Autodesk Inventor part; units mm, degrees
ref_plane "YZ Plane" through (0, 0, 0) normal (1, 0, 0) x (0, 1, 0)
ref_plane "XZ Plane" through (0, 0, 0) normal (0, 1, 0) x (-1, 0, 0)
ref_plane "XY Plane" through (0, 0, 0) normal (0, 0, 1) x (1, 0, 0)
sketch "Sketch1" plane through (0, 0, 0) normal (0, 1, 0) x (-1, 0, 0)
  line L0 (-60, 120) -> (60, 120)
  line L1 (60, 120) -> (60, -110)
  line L2 (50, -120) -> (-50, -120)
  line L3 (-60, -110) -> (-60, 120)
  line L4 (-60, 120) -> (60, -120) construction
  line L5 (60, 120) -> (-60, -120) construction
  line L6 (-60, 120) -> (60, 120)
  line L7 (60, 120) -> (60, 0)
  line L8 (60, 0) -> (-60, 0)
  line L9 (-60, 0) -> (-60, 120)
  line L10 (60, 0) -> (-60, 120) construction
  line L11 (-60, 0) -> (60, 120) construction
  circle A0 centre (0, 60) radius 54
  line L12 (54, 60) -> (60, 60) construction
  arc A1 (50, -120) -> (60, -110) centre (50, -110) ccw
  arc A2 (-60, -110) -> (-50, -120) centre (-50, -110) ccw
  point P0 (0, 0)
  dimension "d0" = 120
  dimension "d1" = 240
  dimension "d2" = 120
  dimension "d3" = 6
  dimension "d4" = 10
extrude "Extrusion1" add sketch "Sketch1" along normal blind 6
sketch "Sketch2" plane through (0, 0, 0) normal (0, -1, 0) x (1, 0, 0)
  circle A0 centre (0, 60) radius 54 construction
  line L0 (60, 120) -> (60, -110)
  line L1 (-60, 120) -> (60, 120)
  line L2 (-60, -110) -> (-60, 120)
  arc A1 (-60, -110) -> (-50, -120) centre (-50, -110) ccw
  line L3 (50, -120) -> (-50, -120)
  arc A2 (50, -120) -> (60, -110) centre (50, -110) ccw
  line L4 (57, -110) -> (57, 117)
  line L5 (57, 117) -> (-57, 117)
  line L6 (-57, 117) -> (-57, -110)
  arc A3 (-57, -110) -> (-50, -117) centre (-50, -110) ccw
  line L7 (-50, -117) -> (50, -117)
  arc A4 (50, -117) -> (57, -110) centre (50, -110) ccw
  line L8 (57, 117) -> (57, 120)
  line L9 (-57, 117) -> (-57, 120)
  point P0 (0, 0)
  dimension "d7" = 3
extrude "Extrusion2" add sketch "Sketch2" along normal blind 15 contours L0 A2 L3 A1 L2 L1 L9 L6 A3 L7 A4 L4 L8
sketch "Sketch3" plane through (0, -15, 0) normal (0, -1, 0) x (1, 0, 0)
  line L0 (60, -110) -> (60, 120)
  line L1 (60, 120) -> (57, 120)
  line L2 (57, 120) -> (57, -110)
  arc A0 (50, -117) -> (57, -110) centre (50, -110) ccw
  line L3 (50, -117) -> (-50, -117)
  arc A1 (-57, -110) -> (-50, -117) centre (-50, -110) ccw
  line L4 (-57, -110) -> (-57, 120)
  line L5 (-57, 120) -> (-60, 120)
  line L6 (-60, 120) -> (-60, -110)
  arc A2 (-60, -110) -> (-50, -120) centre (-50, -110) ccw
  line L7 (-50, -120) -> (50, -120)
  arc A3 (50, -120) -> (60, -110) centre (50, -110) ccw
  line L8 (57, 120) -> (54, 120)
  line L9 (-60, 120) -> (60, 120) construction
  line L10 (54, 120) -> (54, -110)
  line L11 (50, -114) -> (25, -114)
  arc A4 (50, -114) -> (54, -110) centre (50, -110) ccw
  line L12 (0, 0) -> (0, -136) construction
  line L13 (-57, 120) -> (-54, 120)
  line L14 (-54, 120) -> (-54, -110)
  line L15 (-50, -114) -> (25, -114)
  arc A5 (-54, -110) -> (-50, -114) centre (-50, -110) ccw
  dimension "d10" = 3
extrude "Extrusion3" add sketch "Sketch3" along normal blind 6
sketch "Sketch5" plane through (0, 6, 0) normal (0, 1, 0) x (1, 0, 0)
  circle A0 centre (0, -60) radius 54
  line L0 (60, -120) -> (60, 110)
  arc A1 (60, 110) -> (50, 120) centre (50, 110) ccw
  line L1 (50, 120) -> (-50, 120)
  arc A2 (-50, 120) -> (-60, 110) centre (-50, 110) ccw
  line L2 (-60, 110) -> (-60, -120)
  line L3 (-60, -120) -> (60, -120)
  line L4 (-67.6504, 0) -> (67.3496, 0) construction
  circle A3 centre (0, 60) radius 54
  point P0 (0, 0)
extrude "Extrusion4" cut sketch "Sketch5" against normal up to next contours A3
sketch "Sketch6" plane through (0, 6, 0) normal (0, 1, 0) x (1, 0, 0)
  circle A0 centre (0, -60) radius 54
  circle A1 centre (0, 60) radius 54
  circle A2 centre (0, 60) radius 54
  circle A3 centre (0, -60) radius 54
  line L0 (60, -120) -> (60, 110)
  arc A4 (60, 110) -> (50, 120) centre (50, 110) ccw
  line L1 (50, 120) -> (-50, 120)
  arc A5 (-50, 120) -> (-60, 110) centre (-50, 110) ccw
  line L2 (-60, 110) -> (-60, -120)
  line L3 (-60, -120) -> (60, -120)
  line L4 (-50.0326, 0) -> (43.9674, 0) construction
  line L5 (0, -60) -> (-70, -60) construction
  line L6 (0, -60) -> (0, -118) construction
  point P0 (0, 0)
  point P1 (-51, -9)
  point P2 (-51, -111)
  point P3 (51, -9)
  point P4 (51, -111)
  point P5 (-51, 9)
  point P6 (-51, 111)
  point P7 (51, 111)
  point P8 (51, 9)
  dimension "d15" = 18
  dimension "d16" = 9
hole "Hole1" at (-51, 6, 9) at (-51, 6, 111) at (51, 6, 111) at (51, 6, 9) at (-51, 6, -111) at (-51, 6, -9) at (51, 6, -111) at (51, 6, -9) direction (0, -1, 0) diameter 3.1 end through all
sketch "Sketch7" plane through (0, -21, 0) normal (0, -1, 0) x (1, 0, 0)
  line L0 (57, 120) -> (57, -110) construction
  line L1 (57, -110) -> (57, 120)
  line L2 (-57, -110) -> (-57, 120) construction
  line L3 (-57, 120) -> (-57, -110)
  line L4 (57, 120) -> (57, -110)
  line L5 (0, 119) -> (0, 0) construction
  point P0 (57, 60)
  point P1 (57, -60)
  point P2 (57, 114)
  point P3 (-57, 114)
  point P4 (-57, 102)
  point P5 (57, 102)
  point P6 (-57, 90)
  point P7 (57, 90)
  point P8 (-57, 78)
  point P9 (57, 78)
  point P10 (-57, 66)
  point P11 (57, 66)
  point P12 (-57, 54)
  point P13 (57, 54)
  point P14 (-57, 42)
  point P15 (57, 42)
  point P16 (-57, 30)
  point P17 (57, 30)
  point P18 (-57, 18)
  point P19 (57, 18)
  point P20 (-57, 6)
  point P21 (57, 6)
  point P22 (-57, -6)
  point P23 (57, -6)
  point P24 (-57, -18)
  point P25 (57, -18)
  point P26 (-57, -30)
  point P27 (57, -30)
  point P28 (-57, -42)
  point P29 (57, -42)
  point P30 (-57, -54)
  point P31 (57, -54)
  point P32 (-57, -66)
  point P33 (57, -66)
  dimension "d24" = 6
  dimension "d27" = 12
hole "Hole2" at (57, -21, 114) at (-57, -21, 114) at (-57, -21, 102) at (57, -21, 102) at (-57, -21, 90) at (57, -21, 90) at (-57, -21, 78) at (57, -21, 78) at (-57, -21, 66) at (57, -21, 66) at (-57, -21, 54) at (57, -21, 54) at (-57, -21, 42) at (57, -21, 42) at (-57, -21, 30) at (57, -21, 30) at (-57, -21, 18) at (57, -21, 18) at (-57, -21, 6) at (57, -21, 6) at (-57, -21, -6) at (57, -21, -6) at (-57, -21, -18) at (57, -21, -18) at (-57, -21, -30) at (57, -21, -30) at (-57, -21, -42) at (57, -21, -42) at (-57, -21, -54) at (57, -21, -54) at (-57, -21, -66) at (57, -21, -66) direction (0, 1, 0) diameter 3.1 depth 4 tip angle 118
equation "\"d0\" = hull_width"
equation "\"d1\" = hull_length"
equation "\"d2\" = hull_width"
equation "\"d3\" = 2 * thickness"
equation "\"d4\" = roundness"
equation "\"d5\" = 2 * thickness"
equation "\"d7\" = thickness"
equation "\"d8\" = 5 * thickness"
equation "\"d10\" = thickness"
equation "\"d11\" = 2 * thickness"
equation "\"d13\" = 2 * thickness"
equation "\"d22\" = 1.33333 * thickness"
equation "\"d37\" = 1.33333 * thickness"
equation "\"thickness\" = 3"
equation "\"roundness\" = 10"
equation "\"hull_width\" = 120"
equation "\"hull_length\" = 2 * hull_width"
properties part number "Cup_Dispenser_Hull"
Here's how the part is built. I have some questions about the finished solid (model axes, mm). A direction names the side the tool comes from. Round coordinates to 2 decimals unless told otherwise and drop trailing zeros. Order: outer loops, then holes, each group sorted by start corner. A loop starts at its lowest first (then second) coordinate and runs counter-clockwise, first axis right, second up. Notation, with made-up numbers: (-29, 31.5) -> (0, 31.5) arc R29 ccw to (0, 63.5) -> close; hole circle Ø9 at (24, 50.5). An arc over 180 degrees is marked (long way). Use a Markdown table: item, result. Add a question column.
(1) For faces 4 (the face through (-57, -7, 3)), 5 (the face through (-56.99, -7.31, -117.15)), 6 (the face through (-54, -18, 7)), which set-ups out of +Z, -Z, +X, -X, +Y, -Y let a thin tool reach every point of the face, with its end or its side?
(2) Suppose I cut it at C-C, the plane x = -16. Please give me the cut outline in (y, z), and give its area (3 significant figures).
(3) Suppose I cut it at A-A, the plane x = 35. Please give me the cut outline in (y, z), and give its area (3 significant figures).
(4) Suppose I cut it at B-B, the plane y = -9.75. Please give me the cut outline in (x, z), and give its area (3 significant figures).
(5) I need wall thicknesses on line 1 along X through (y, z) = (-20, -54); line 2 along X through (y, z) = (-12.5, 65); line 3 along X through (y, z) = (-19.5, 3). Which ranges of each line are inside material? Lowest first, please.
(6) For pin 1 Ø3.5 at (x, z) = (-51, 9) entering from -Y; pin 2 Ø1.5 at (x, y) = (-3, -6) entering from +Z; pin 3 Ø1.9 at (x, z) = (51, 9) entering from -Y; pin 4 Ø2.5 at (x, z) = (-57, 90) entering from -Y, each with a flat end and sliding along its axis, tell me the tip position at first contact or that it passes through.
(7) If we mould it in two halves opening along X, with no side actions, what happens to faces 1 (the face through (1, -7, -120)), 2 (the face through (57.15, -7.31, -116.99)), 3 (the face through (-54.9, -7.4, -115))? For each: released by +X, released by -X, zero draft, split by the parting line, or undercut.
Verdict:
| question | item | result |
|---|---|---|
| 1 | face 4 | +Z |
| 1 | face 5 | -Z, -X, +Y, -Y |
| 1 | face 6 | +Z, -Y |
| 2 | outline | (-21, -120) -> (6, -120) -> (6, -111.58) -> (0, -111.58) -> (0, -117) -> (-15, -117) -> (-15, -114) -> (-21, -114) -> close; (0, -8.42) -> (6, -8.42) -> (6, 8.42) -> (0, 8.42) -> close; (0, 111.58) -> (6, 111.58) -> (6, 120) -> (0, 120) -> close |
| 2 | area | 283 mm2 |
| 3 | outline | (-21, -120) -> (6, -120) -> (6, -101.12) -> (0, -101.12) -> (0, -117) -> (-15, -117) -> (-15, -114) -> (-21, -114) -> close; (0, -18.88) -> (6, -18.88) -> (6, 18.88) -> (0, 18.88) -> close; (0, 101.12) -> (6, 101.12) -> (6, 120) -> (0, 120) -> close |
| 3 | area | 534 mm2 |
| 4 | outline | (-60, -110) arc R10 ccw to (-50, -120) -> (50, -120) arc R10 ccw to (60, -110) -> (60, 120) -> (57, 120) -> (57, -110) arc R7 cw to (50, -117) -> (-50, -117) arc R7 cw to (-57, -110) -> (-57, 120) -> (-60, 120) -> close |
| 4 | area | 1,760 mm2 |
| 5 | line 1 | -60 to -58.55, -55.45 to -54, 54 to 55.45, 58.55 to 60 |
| 5 | line 2 | -60 to -57, 57 to 60 |
| 5 | line 3 | -60 to -54, 54 to 60 |
| 6 | pin 1 | y = 0 |
| 6 | pin 2 | z = -117 |
| 6 | pin 3 | through |
| 6 | pin 4 | y = -16.82 |
| 7 | face 1 | zero draft |
| 7 | face 2 | released by +X |
| 7 | face 3 | undercut |
